```python
from build123d import *

# Parameters (mm, degrees)
EXTRUDE_1_DEPTH     = 10
SKETCH_2_R          = 1.75
CUT_EXTRUDE_1_DEPTH = 32.463731502
SKETCH_3_W          = 10
SKETCH_3_H          = 15.5
EXTRUDE_2_DEPTH     = 10
SKETCH_4_R          = 3.2
CUT_EXTRUDE_2_DEPTH = 2.6
SKETCH_5_R          = 1
CUT_EXTRUDE_3_DEPTH = 34.631367799
FILLET_1_R          = 3
FILLET_2_R          = 3
CHAMFER_1_SIZE      = 0.6
FILLET_3_R          = 7.5


# Some blends are built 0.0001 mm under size
with BuildPart() as part:
    # ｽｹｯﾁ1 → ﾎﾞｽ - 押し出し1 (new body)
    with BuildSketch(Plane(origin=(0, 0, 0), x_dir=(1, 0, 0), z_dir=(0, 1, 0))):
        Polygon((-15.1, -8.2), (5.1, -8.2), (5.1, -5.2), (-5.1, -5.2), (-5.1, 5.2), (5.1, 5.2), (5.1, 8.2), (-15.1, 8.2), align=None)
        Polygon((-15.1, -8.2), (-15.1, -4.75), (-24.92, -4.75), (-24.92, -20.25), (-14.92, -20.25), (-14.92, -8.2), align=None)
    extrude(amount=EXTRUDE_1_DEPTH)

    # ｽｹｯﾁ2 → ｶｯﾄ - 押し出し1 (cut, through all)
    with BuildSketch(Plane.XY.offset(8.2)):
        with Locations((0, 5)):
            Circle(SKETCH_2_R)
    extrude(amount=-CUT_EXTRUDE_1_DEPTH, mode=Mode.SUBTRACT)

    # ｽｹｯﾁ3 → ﾎﾞｽ - 押し出し2 (add)
    with BuildSketch(Plane(origin=(0, 10, 0), x_dir=(1, 0, 0), z_dir=(0, 1, 0))):
        with Locations((-19.92, -12.5)):
            Rectangle(SKETCH_3_W, SKETCH_3_H)
    extrude(amount=EXTRUDE_2_DEPTH)

    # ｽｹｯﾁ4 → ｶｯﾄ - 押し出し2 (cut)
    with BuildSketch(Plane(origin=(0, 20, 0), x_dir=(1, 0, 0), z_dir=(0, 1, 0))):
        with Locations(Location((-19.92, -12.5, 0), (0, 0, 270))):
            Circle(SKETCH_4_R)
    extrude(amount=-CUT_EXTRUDE_2_DEPTH, mode=Mode.SUBTRACT)

    # ｽｹｯﾁ5 → ｶｯﾄ - 押し出し3 (cut, through all)
    with BuildSketch(Plane(origin=(0, 10, 0), x_dir=(1, 0, 0), z_dir=(0, 1, 0))):
        with Locations((-5.1, 5.2)):
            Circle(SKETCH_5_R)
        with Locations((-5.1, -5.2)):
            Circle(SKETCH_5_R)
    extrude(amount=-CUT_EXTRUDE_3_DEPTH, mode=Mode.SUBTRACT)

    # ﾌｨﾚｯﾄ1
    fillet_1_edges = [part.edges().sort_by_distance(p)[0] for p in [
        (-14.92, 10, 20.25),
        (-24.92, 10, 20.25),
        (-24.92, 10, 4.75),
        (-15.1, 5, 4.75),
        (5.1, 5, -8.2),
        (5.1, 5, 8.2),
        (-14.92, 10, 6.475),
        (-14.92, 5, 8.2),
    ]]
    fillet(fillet_1_edges, radius=FILLET_1_R - 0.0001)  # a hair under: the kernel refuses the full size

    # ﾌｨﾚｯﾄ2
    fillet_2_edges = [part.edges().sort_by_distance(p)[0] for p in [
        (-15.01, 10, 4.75),
    ]]
    fillet(fillet_2_edges, radius=FILLET_2_R - 0.0001)  # a hair under: the kernel refuses the full size

    # 面取り1
    # the kernel refuses this chamfer: 0.6 mm, written as the material it takes off along each edge
    with BuildSketch(Plane(origin=(-18.0999, 0, 1.7501), x_dir=(0, 0, 1), z_dir=(-1, 0, 0))) as chamfer_1_piece_1:
        Polygon((2.9999, CHAMFER_1_SIZE), (2.9999 + CHAMFER_1_SIZE, 0), (2.9999, 0), align=None)
    revolve(axis=Axis((-18.0999, 0, 1.7501), (0, 1, 0)), revolution_arc=90, mode=Mode.SUBTRACT)
    with BuildSketch(Plane(origin=(-11.9201, 0, 11.1999), x_dir=(0, 0, -1), z_dir=(1, 0, 0))) as chamfer_1_piece_2:
        Polygon((2.9999, CHAMFER_1_SIZE), (2.9999 + CHAMFER_1_SIZE, 0), (2.9999, 0), align=None)
    revolve(axis=Axis((-11.9201, 0, 11.1999), (0, 1, 0)), revolution_arc=90, mode=Mode.SUBTRACT)
    with BuildSketch(Plane(origin=(-15.1, 0, -9.743009793), x_dir=(-0.027495876610587354, 0.9996219169112968, 0), z_dir=(0, 0, 1))) as chamfer_1_piece_3:
        Polygon((CHAMFER_1_SIZE * 0.999621916911, -CHAMFER_1_SIZE * 0.0274958766106), (-CHAMFER_1_SIZE * 0.0274958766106, -CHAMFER_1_SIZE * 0.999621916911), (0, 0), align=None)
    extrude(amount=11.493109793, mode=Mode.SUBTRACT)
    with BuildSketch(Plane(origin=(-5.643009793, 0, -5.2), x_dir=(0, 0.9996219169112968, 0.027495876610585914), z_dir=(1, 0, 0)), Plane(origin=(6.643009793, 0, 5.2), x_dir=(0, 0.9996219169112968, -0.027495876610585914), z_dir=(-1, 0, 0))) as chamfer_1_piece_4:
        Polygon((CHAMFER_1_SIZE * 0.999621916911, -CHAMFER_1_SIZE * 0.0274958766106), (-CHAMFER_1_SIZE * 0.0274958766106, -CHAMFER_1_SIZE * 0.999621916911), (0, 0), align=None)
    extrude(amount=12.286019586, mode=Mode.SUBTRACT)
    with BuildSketch(Plane(origin=(-5.1, 0, 5.743009793), x_dir=(0.027495876610585914, 0.9996219169112968, 0), z_dir=(0, 0, -1))) as chamfer_1_piece_5:
        Polygon((CHAMFER_1_SIZE * 0.999621916911, -CHAMFER_1_SIZE * 0.0274958766106), (-CHAMFER_1_SIZE * 0.0274958766106, -CHAMFER_1_SIZE * 0.999621916911), (0, 0), align=None)
    extrude(amount=11.486019586, mode=Mode.SUBTRACT)
    with BuildSketch(Plane(origin=(-5.1, 0, 5.2), x_dir=(0.7048818539423609, 0, -0.7093247295722744), z_dir=(0.7093247295722744, 0, 0.7048818539423609))) as chamfer_1_piece_6:
        Polygon((1, CHAMFER_1_SIZE), (1 + CHAMFER_1_SIZE, 0), (1, 0), align=None)
    revolve(axis=Axis((-5.1, 0, 5.2), (0, 1, 0)), revolution_arc=359.64, mode=Mode.SUBTRACT)
    with BuildSketch(Plane(origin=(-5.1, 0, -5.2), x_dir=(0.7093247295722735, 0, 0.7048818539423618), z_dir=(-0.7048818539423618, 0, 0.7093247295722735))) as chamfer_1_piece_7:
        Polygon((1, CHAMFER_1_SIZE), (1 + CHAMFER_1_SIZE, 0), (1, 0), align=None)
    revolve(axis=Axis((-5.1, 0, -5.2), (0, 1, 0)), revolution_arc=359.64, mode=Mode.SUBTRACT)
    with BuildSketch(Plane(origin=(-14.92, 0, 17.2501), x_dir=(0.027495876610587354, 0.9996219169112968, 0), z_dir=(0, 0, -1))) as chamfer_1_piece_8:
        Polygon((CHAMFER_1_SIZE * 0.999621916911, -CHAMFER_1_SIZE * 0.0274958766106), (-CHAMFER_1_SIZE * 0.0274958766106, -CHAMFER_1_SIZE * 0.999621916911), (0, 0), align=None)
    extrude(amount=6.0502, mode=Mode.SUBTRACT)
    with BuildSketch(Plane(origin=(-11.9201, 0, 8.2), x_dir=(0, 0.9996219169112968, 0.027495876610587354), z_dir=(1, 0, 0))) as chamfer_1_piece_9:
        Polygon((CHAMFER_1_SIZE * 0.999621916911, -CHAMFER_1_SIZE * 0.0274958766106), (-CHAMFER_1_SIZE * 0.0274958766106, -CHAMFER_1_SIZE * 0.999621916911), (0, 0), align=None)
    extrude(amount=14.0202, mode=Mode.SUBTRACT)
    with BuildSketch(Plane(origin=(-21.9201, 0, 20.25), x_dir=(0, 0.9996219169112968, 0.027495876610584478), z_dir=(1, 0, 0))) as chamfer_1_piece_10:
        Polygon((CHAMFER_1_SIZE * 0.999621916911, -CHAMFER_1_SIZE * 0.0274958766106), (-CHAMFER_1_SIZE * 0.0274958766106, -CHAMFER_1_SIZE * 0.999621916911), (0, 0), align=None)
    extrude(amount=4.0002, mode=Mode.SUBTRACT)
    with BuildSketch(Plane(origin=(-24.92, 0, 7.7499), x_dir=(-0.027495876610584478, 0.9996219169112968, 0), z_dir=(0, 0, 1))) as chamfer_1_piece_11:
        Polygon((CHAMFER_1_SIZE * 0.999621916911, -CHAMFER_1_SIZE * 0.0274958766106), (-CHAMFER_1_SIZE * 0.0274958766106, -CHAMFER_1_SIZE * 0.999621916911), (0, 0), align=None)
    extrude(amount=9.5002, mode=Mode.SUBTRACT)
    with BuildSketch(Plane(origin=(-18.0999, 0, 4.75), x_dir=(0, -0.02749587661058641, 0.9996219169112968), z_dir=(-1, 0, 0))) as chamfer_1_piece_12:
        Polygon((CHAMFER_1_SIZE * 0.999621916911, CHAMFER_1_SIZE * 0.0274958766106), (-CHAMFER_1_SIZE * 0.0274958766106, CHAMFER_1_SIZE * 0.999621916911), (0, 0), align=None)
    extrude(amount=3.8202, mode=Mode.SUBTRACT)
    with BuildSketch(Plane(origin=(2.1001, 0, -8.2), x_dir=(0, 0.9996219169112968, -0.027495876610587354), z_dir=(-1, 0, 0))) as chamfer_1_piece_13:
        Polygon((CHAMFER_1_SIZE * 0.999621916911, -CHAMFER_1_SIZE * 0.0274958766106), (-CHAMFER_1_SIZE * 0.0274958766106, -CHAMFER_1_SIZE * 0.999621916911), (0, 0), align=None)
    extrude(amount=18.743109793, mode=Mode.SUBTRACT)
    with BuildSketch(Plane(origin=(2.1001, 0, 5.2001), x_dir=(0, 0, 1), z_dir=(-1, 0, 0))) as chamfer_1_piece_14:
        Polygon((2.9999, CHAMFER_1_SIZE), (2.9999 - CHAMFER_1_SIZE, 0), (2.9999, 0), align=None)
    revolve(axis=Axis((2.1001, 0, 5.2001), (0, 1, 0)), revolution_arc=90, mode=Mode.SUBTRACT)
    with BuildSketch(Plane(origin=(2.1001, 0, -5.2001), x_dir=(0, 0, -1), z_dir=(-1, 0, 0))) as chamfer_1_piece_15:
        Polygon((2.9999, -CHAMFER_1_SIZE), (2.9999 - CHAMFER_1_SIZE, 0), (2.9999, 0), align=None)
    revolve(axis=Axis((2.1001, 0, -5.2001), (0, -1, 0)), revolution_arc=90, mode=Mode.SUBTRACT)
    with BuildSketch(Plane(origin=(-21.9201, 0, 7.7499), x_dir=(-1, 0, 0), z_dir=(0, 0, 1))) as chamfer_1_piece_16:
        Polygon((2.9999, -CHAMFER_1_SIZE), (2.9999 - CHAMFER_1_SIZE, 0), (2.9999, 0), align=None)
    revolve(axis=Axis((-21.9201, 0, 7.7499), (0, -1, 0)), revolution_arc=90, mode=Mode.SUBTRACT)
    with BuildSketch(Plane(origin=(-21.9201, 0, 17.2501), x_dir=(0, 0, 1), z_dir=(1, 0, 0))) as chamfer_1_piece_17:
        Polygon((2.9999, -CHAMFER_1_SIZE), (2.9999 - CHAMFER_1_SIZE, 0), (2.9999, 0), align=None)
    revolve(axis=Axis((-21.9201, 0, 17.2501), (0, -1, 0)), revolution_arc=90, mode=Mode.SUBTRACT)
    with BuildSketch(Plane(origin=(-17.9199, 0, 17.2501), x_dir=(1, 0, 0), z_dir=(0, 0, -1))) as chamfer_1_piece_18:
        Polygon((2.9999, -CHAMFER_1_SIZE), (2.9999 - CHAMFER_1_SIZE, 0), (2.9999, 0), align=None)
    revolve(axis=Axis((-17.9199, 0, 17.2501), (0, -1, 0)), revolution_arc=90, mode=Mode.SUBTRACT)
    with BuildSketch(Plane(origin=(5.1, 0, -3.656990207), x_dir=(0.027495876610585918, 0.9996219169112968, 0), z_dir=(0, 0, -1)), Plane(origin=(5.1, 0, 5.2001), x_dir=(0.027495876610585918, 0.9996219169112968, 0), z_dir=(0, 0, -1))) as chamfer_1_piece_19:
        Polygon((CHAMFER_1_SIZE * 0.999621916911, -CHAMFER_1_SIZE * 0.0274958766106), (-CHAMFER_1_SIZE * 0.0274958766106, -CHAMFER_1_SIZE * 0.999621916911), (0, 0), align=None)
    extrude(amount=1.543109793, mode=Mode.SUBTRACT)

    # ﾌｨﾚｯﾄ3
    # the kernel refuses this fillet: 7.5 mm, written as the material it takes off along each edge
    with BuildSketch(Plane(origin=(-15.1, -18.15, -8.2), x_dir=(0, 0, 1), z_dir=(0, 1, 0))) as fillet_3_piece_1:
        with BuildLine():
            CenterArc((FILLET_3_R, FILLET_3_R), FILLET_3_R, 180, 90)
            Line((0, FILLET_3_R), (0, 0))
            Line((0, 0), (FILLET_3_R, 0))
        make_face()
    extrude(amount=46.9, mode=Mode.SUBTRACT)


solid = part.part
```
Can you work these out from the model? Positions are in its coordinate system, mm. A direction names the side the tool comes from. Round coordinates to 2 decimals unless told otherwise and drop trailing zeros. Loops run counter-clockwise (first coordinate to the right, second up) from the corner with the lowest first, then second, coordinate; pieces in that order, holes last. Notation, with made-up numbers: M 36,37 L 56,37 A12 ccw 56,59 Z; hole C 39.5,15 d1. An arc over 180 degrees is marked long. Write item = value, one per line. Start each with the question number.
(1) I'm going to push flat-ended pins straight in: P1, Ø3, axis at x = 1, y = 4.5, coming from the +Z side; P2, Ø12, axis at x = -10.5, z = 12, coming from the -Y side; P3, Ø1.5, axis at x = -14.5, y = 17, coming from the -Z side; P4, Ø2.5, axis at y = 7, z = 0, coming from the -X side. Where does each tip first touch, or does it pass through?
(2) Suppose I cut it at B-B on y = 5. Give the number of separate pieces and of enclosed holes in the cut face, plus the area to 3 significant figures.
(3) If we mould it in two halves opening along Z, with no side actions, what happens to faces 1 (the face through (-12.845, 4.93, -6.061)), 2 (the face through (-7, 10, 0)), 3 (the face through (-5.783, 5.366, -5.93))? For each: released by +Z, released by -Z, zero draft, split by the parting line, or undercut.
(4) Suppose I cut it at A-A on x = 0. Write out the boundary of the cut face in (y, z), plus the area to 3 significant figures.
(5) I need wall thicknesses on line 1 along X through (y, z) = (19.25, 12.5); line 2 along Z through (x, y) = (-21, 13.75); line 3 along X through (y, z) = (11.25, 15.5). Which ranges of each line are inside material? Lowest first, please.
(6) Suppose I cut it at C-C on z = 12.5. Write out the boundary of the cut face in (x, y), plus the area to 3 significant figures.
(7) Which directions (+Z, -Z, +X, -X, +Y, -Y) give clear straight access to the entire face, cutting with the end or side of a thin tool? Please do faces 4 (the face through (-24.06, 10.44, 19.35)), 5 (the face through (-15.1, 5, 1)), 6 (the face through (-20, 17.4, 12)), 7 (the face through (-19, 12, 4.75)).
(8) Suppose I cut it at D-D on y = 13.5. Write out the boundary of the cut face in (x, z), plus the area to 3 significant figures.
Answer block:
q1.P1 = 8.2
q1.P2 = 0
q1.P3 = 4.75
q1.P4 = -15.1
q2.separate_pieces = 3
q2.enclosed_holes = 0
q2.area = 336 mm²
q3.face_1 = released by -Z
q3.face_2 = zero draft
q3.face_3 = undercut
q4.outline = M 0,-7.6 L 0.6,-8.2 L 3.25,-8.2 L 3.25,-5.2 L 0.6,-5.2 L 0,-5.8 Z; M 0,5.8 L 0.6,5.2 L 3.25,5.2 L 3.25,8.2 L 0.6,8.2 L 0,7.6 Z; M 6.75,-8.2 L 10,-8.2 L 10,-5.2 L 6.75,-5.2 Z; M 6.75,5.2 L 10,5.2 L 10,8.2 L 6.75,8.2 Z
q4.area = 38.3 mm²
q5.line_1 = -24.92 to -23.12, -16.72 to -14.92
q5.line_2 = 4.75 to 20.25
q5.line_3 = -24.92 to -14.92
q6.outline = M -24.92,0.6 L -24.32,0 L -15.52,0 L -14.92,0.6 L -14.92,20 L -16.72,20 L -16.72,17.4 L -23.12,17.4 L -23.12,20 L -24.92,20 Z
q6.area = 183 mm²
q7.face_4 = +Z, -X, +Y, -Y
q7.face_5 = -Z, -X, +Y, -Y
q7.face_6 = +Y
q7.face_7 = -Z, -X, +Y
q8.outline = M -24.92,7.75 A3 ccw -21.92,4.75 L -14.92,4.75 L -14.92,17.25 A3 ccw -17.92,20.25 L -21.92,20.25 A3 ccw -24.92,17.25 Z
q8.area = 149 mm²
